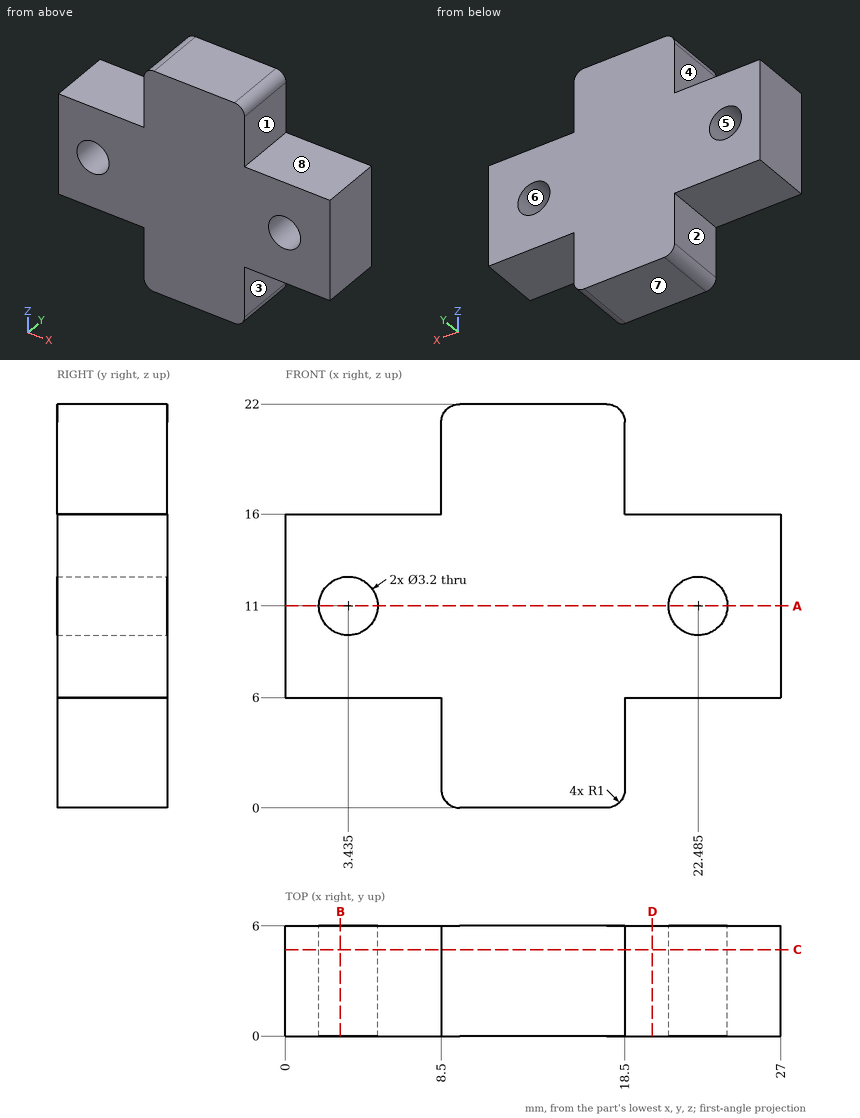
Verification items for this drawing (mm, ordinates from the low corner). A direction names the side the tool comes from. Coordinates: 2 decimals unless noted, no trailing zeros. Write each loop counter-clockwise with the first axis right and the second up, starting at its lowest first coordinate (ties: lowest second). Pieces come first, ordered by that corner, then holes. Notation, with made-up numbers: M 63.25,74 L 86.25,74 A19 ccw 86.25,98 Z; hole C 10,82.25 d2. An arc over 180 degrees is marked long. One line per item, written item: value. Start each with the question number.
(1) Release check for a two-part mould opening along Z. For the marked faces 5, 6, 7 and 8 record: released by +Z, released by -Z, zero draft, split by the parting line, or undercut.
(2) Depth check by flat-ended pin: pin 1 (2.5 mm diameter, centred on y = 4.5, z = 19, fed in from -X); pin 2 (3 mm diameter, centred on x = 23.5, y = 4, fed in from +Z); pin 3 (2.5 mm diameter, centred on y = 3, z = 2.5, fed in from +X). Enter the tip coordinate at first touch or a pass-through.
(3) Sectioned sample at C-C, the plane y = 4.7. Enter the section's corners in (x, z) (3 decimals).
(4) Sectioned sample at A-A, the plane z = 11. Enter the section's corners in (x, y) (3 decimals).
(5) Sectioned sample at D-D, the plane x = 20. Enter the section's corners in (y, z), and give its area (3 significant figures).
(6) Scan lines: line 1 along X through (y, z) = (2.25, 11) (3 decimals); line 2 along X through (y, z) = (3.8, 3.5); line 3 along Z through (x, y) = (19.75, 0.8). Record each from-to range of solid material in increasing order. Write a range as [from, to].
(7) Sectioned sample at B-B, the plane x = 3. Enter the section's corners in (y, z), and give its area (3 significant figures).
(8) Tool access check on the marked faces 1, 2, 3 and 4. Record the directions out of +Z, -Z, +X, -X, +Y, -Y that give a thin tool (end or side, any length) a straight path to the whole face; none if there is none.
Filled sheet:
1. face 5: undercut
1. face 6: undercut
1. face 7: released by -Z
1. face 8: released by +Z
2. pin 1: x = 8.5
2. pin 2: z = 16
2. pin 3: x = 18.5
3. outline: M 0,6 L 8.5,6 L 8.5,1 A1 ccw 9.5,0 L 17.5,0 A1 ccw 18.5,1 L 18.5,6 L 27,6 L 27,16 L 18.5,16 L 18.5,21 A1 ccw 17.5,22 L 9.5,22 A1 ccw 8.5,21 L 8.5,16 L 0,16 Z; hole C 3.435,11 d3.2; hole C 22.485,11 d3.2
4. outline: M 0,0 L 1.835,0 L 1.835,6 L 0,6 Z; M 5.035,0 L 20.885,0 L 20.885,6 L 5.035,6 Z; M 24.085,0 L 27,0 L 27,6 L 24.085,6 Z
5. outline: M 0,6 L 6,6 L 6,16 L 0,16 Z
5. area: 60.0 mm²
6. line 1: [0, 1.835], [5.035, 20.885], [24.085, 27]
6. line 2: [8.5, 18.5]
6. line 3: [6, 16]
7. outline: M 0,6 L 6,6 L 6,9.46 L 0,9.46 Z; M 0,12.54 L 6,12.54 L 6,16 L 0,16 Z
7. area: 41.5 mm²
8. face 1: +Z, +X, +Y, -Y
8. face 2: -Z, -X, +Y, -Y
8. face 3: -Z, +X, +Y, -Y
8. face 4: +Z, -X, +Y, -Y
